Source: CAD feature listing. Evaluate the final solid. Frame: model axes, mm. A direction names the side the tool comes from. Coordinates: 2 decimals unless noted, no trailing zeros. Loops run counter-clockwise (first coordinate to the right, second up) from the corner with the lowest first, then second, coordinate; pieces in that order, holes last.
Item 1: Pull-direction query (X, two-part tool) for faces 1 (the cylindrical face through (7.68, -20.24, 1.6)), 2 (the flat face through (8, -16, 0)), 3 (the cylindrical face through (8.288, -3.444, 0.113)), 4 (the cylindrical face through (0.3, -31.2, 4)); classes: +X half, -X half, draft (parallel to the pull), parting line (faces both ways), or undercut.
Item 2: Line query: probe 1 along X at (y, z) = (-9.5, 2.5) (3 decimals); probe 2 along Y at (x, z) = (7.75, 1.25); probe 3 along Y at (x, z) = (7.25, 3). Output: solid intervals per line, ascending.
Item 3: Reachability of faces 5 (the flat face through (5, -23, 3.25)), 6 (the flat face through (8.33, -28.42, 1.53)) from +Z, -Z, +X, -X, +Y, -Y: full face, straight path, thin tool, end or side. Return the list, or none.
Item 4: Section query C-C, the plane y = -18.5. Return the cut outline in (x, z) (3 decimals).
Item 5: Pin query (flat end, axial travel): pin 1 Ø1.5 at (x, z) = (2.5, 3) entering from +Y; pin 2 Ø3 at (x, z) = (11.5, 4.5) entering from -Y; pin 3 Ø4.5 at (y, z) = (-25, 5.5) entering from +X (3 decimals); pin 4 Ø4 at (x, y) = (9, -25.5) entering from +Z. Return the tip coordinate at first contact, or that it passes through.
Item 6: Section query A-A, the plane y = -8.5. Return the cut outline in (x, z) (3 decimals).
Item 7: Section query D-D, the plane z = 2.5. Return the cut outline in (x, y) (1 decimal), then the cut area to 3 significant figures.
```python
from build123d import *

# Parameters (mm, degrees)
SKETCH1_R           = 2
BOSS_EXTRUDE1_DEPTH = 7.5
FILLET1_R           = 0.79375
CUT_EXTRUDE1_DEPTH  = 4.25
FILLET2_R           = 0.396875


with BuildPart() as part:
    # Sketch1 → Boss-Extrude1 (new body)
    with BuildSketch(Plane.XY):
        Polygon((0, 0), (15.875, -6.35), (15.875, -25.4), (0, -31.75), align=None)
        with Locations((7.9375, -22.225)):
            Circle(SKETCH1_R, mode=Mode.SUBTRACT)
        with Locations((7.9375, -9.525)):
            Circle(SKETCH1_R, mode=Mode.SUBTRACT)
    extrude(amount=BOSS_EXTRUDE1_DEPTH)

    # Fillet1
    fillet1_edges = [part.edges().sort_by_distance(p)[0] for p in [
        (0, 0, 3.75),
        (15.875, -6.35, 3.75),
        (15.875, -25.4, 3.75),
        (0, -31.75, 3.75),
    ]]
    fillet(fillet1_edges, radius=FILLET1_R)

    # Sketch2 → Cut-Extrude1 (cut)
    with BuildSketch(Plane.XY.offset(7.5)):
        with BuildLine():
            Line((14.6875, -22.225), (14.6875, -25.875))
            Line((14.6875, -25.875), (1.1875, -31.275))
            Line((1.1875, -31.275), (1.1875, -22.225))
            ThreePointArc((1.1875, -22.225), (7.9375, -15.475), (14.6875, -22.225))
        make_face()
    extrude(amount=-CUT_EXTRUDE1_DEPTH, mode=Mode.SUBTRACT)

    # Fillet2
    fillet2_edges = [part.edges().sort_by_distance(p)[0] for p in [
        (8.232291349, -28.45708346, 0),
        (0, -15.875, 0),
        (8.232291349, -3.29291654, 0),
        (15.875, -15.875, 0),
        (0.348750883, -0.515116549, 0),
        (15.738528364, -6.442395796, 0),
        (15.738528364, -25.307604204, 0),
        (0.348750883, -31.234883451, 0),
    ]]
    fillet(fillet2_edges, radius=FILLET2_R)


solid = part.part
```
Verdict:
1. face 1: undercut
1. face 2: draft
1. face 3: +X half
1. face 4: parting line
2. probe 1: x = 0 to 5.938, 9.937 to 15.875
2. probe 2: y = -28.65 to -24.22, -20.23 to -11.52, -7.53 to -3.1
2. probe 3: y = -28.85 to -24.1, -20.35 to -11.4, -7.65 to -2.9
3. face 5: +Z, -Y
3. face 6: +Z, -Z, +X, -Y
4. outline: (0, 0.397) arc R0.397 ccw to (0.397, 0) - (15.478, 0) arc R0.397 ccw to (15.875, 0.397) - (15.875, 7.5) - (13.567, 7.5) - (13.567, 3.25) - (2.308, 3.25) - (2.308, 7.5) - (0, 7.5) - close
5. pin 1: stops at y = -0.7
5. pin 2: stops at y = -27.48
5. pin 3: stops at x = 15.875
5. pin 4: stops at z = 3.25
6. outline: (0, 0.397) arc R0.397 ccw to (0.397, 0) - (6.22, 0) - (6.22, 7.5) - (0, 7.5) - close; (9.655, 0) - (15.478, 0) arc R0.397 ccw to (15.875, 0.397) - (15.875, 7.5) - (9.655, 7.5) - close
7. outline: (0, -30.6) arc R0.8 ccw to (1.1, -31.3) - (15.4, -25.6) arc R0.8 ccw to (15.9, -24.9) - (15.9, -6.9) arc R0.8 ccw to (15.4, -6.2) - (1.1, -0.4) arc R0.8 ccw to (0, -1.2) - close; hole circle Ø4 at (7.9, -22.2); hole circle Ø4 at (7.9, -9.5)
7. area: 377 mm2
